```python
from build123d import *

# Parameters (mm, degrees)
F0_R     = 4.05
F0_R_2   = 3.4
F0_R_3   = 5.5
F1_DEPTH = 1.5
F2_DEPTH = 9.2
F3_DEPTH = 9.201
F4_SIZE  = 0.3


with BuildPart() as f1:
    # F0 (on Right) → F1 (new body)
    with BuildSketch(Plane.YZ):
        Circle(F0_R)
        Circle(F0_R_2, mode=Mode.SUBTRACT)
        Circle(F0_R_2)
        Circle(F0_R_3)
        Circle(F0_R, mode=Mode.SUBTRACT)
    extrude(amount=F1_DEPTH)

    # F0 (on Right) → F2 (join)
    with BuildSketch(Plane.YZ):
        Circle(F0_R)
        Circle(F0_R_2, mode=Mode.SUBTRACT)
    extrude(amount=F2_DEPTH)

    # F0 (on Right) → F3 (cut, through all)
    with BuildSketch(Plane.YZ):
        Circle(F0_R_2)
    extrude(amount=F3_DEPTH, mode=Mode.SUBTRACT)

    # F4
    f4_edges = [f1.edges().sort_by_distance(p)[0] for p in [
        (0, -3.4, 0),
        (9.2, -4.05, 0),
    ]]
    chamfer(f4_edges, length=F4_SIZE)


solid = f1.part
```
Work out the finished part from the listing and answer in its coordinate system (mm). Round coordinates to 2 decimals unless told otherwise and drop trailing zeros. Order: outer loops, then holes, each group sorted by start corner. A loop starts at its lowest first (then second) coordinate and runs counter-clockwise, first axis right, second up.
Q1. Find the intervals of material crossed by line 1 along Z through (x, y) = (3, 0); line 2 along X through (y, z) = (-4.25, -0.5); line 3 along Z through (x, y) = (7.5, 3), in increasing order.
Solution:
line 1: z = -4.05 to -3.4, 3.4 to 4.05
line 2: x = 0 to 1.5
line 3: z = -2.72 to -1.6, 1.6 to 2.72
Q2. The mould has two halves that part along Y. Classify faces 1 (the flat face through (0, 4, -1)), 2 (the cylindrical face through (0.74, -1.19, -5.37)), 3 (the cylindrical face through (4.69, -0.74, -3.32)): pulls with the +Y half, pulls with the -Y half, needs draft (parallel to the pull), parting line crosses it, or undercut.
Solution:
face 1: needs draft
face 2: parting line crosses it
face 3: undercut
Q3. A cutting plane is placed at C-C, the plane x = 7. Determine the outline of the cut face in (y, z).
Solution:
outline: circle Ø8.1 at (0, 0); hole circle Ø6.8 at (0, 0)
Q4. Given pin 1 Ø4 at (x, y) = (8, -2) entering from +Z; pin 2 Ø1.5 at (y, z) = (2.5, -1) entering from -X; pin 3 Ø5 at (x, z) = (2.5, -3.5) entering from +Y, each flat-ended and moving along its own axis, determine where each tip first touches the part or whether it passes through.
Solution:
pin 1: stops at z = 4.05
pin 2: stops at x = 0.26
pin 3: stops at y = 5.37
Q5. A cutting plane is placed at A-A, the plane z = 0. Determine the outline of the cut face in (x, y).
Solution:
outline: (0, -5.5) - (1.5, -5.5) - (1.5, -4.05) - (8.9, -4.05) - (9.2, -3.75) - (9.2, -3.4) - (0.3, -3.4) - (0, -3.7) - close; (0, 3.7) - (0.3, 3.4) - (9.2, 3.4) - (9.2, 3.75) - (8.9, 4.05) - (1.5, 4.05) - (1.5, 5.5) - (0, 5.5) - close
